Model file for the job. Use its own axes, mm. A direction names the side the tool comes from. Coordinates: 2 decimals unless noted, no trailing zeros. Loops run counter-clockwise (first coordinate to the right, second up) from the corner with the lowest first, then second, coordinate; pieces in that order, holes last.
from build123d import *

# Parameters (mm, degrees)
SKETCH2_W           = 10
SKETCH2_H           = 30
BOSS_EXTRUDE1_DEPTH = 2


with BuildPart() as part:
    # Sketch2 → Boss-Extrude1 (new body)
    with BuildSketch(Plane.XY):
        with Locations((10, -15)):
            Rectangle(SKETCH2_W, SKETCH2_H)
        Polygon((0, 7), (0, 0), (5, 0), (15, 0), (16.8, 0), (16.8, 2.1), (7.2, 4.9), align=None)
        Polygon((8.6, 9.7), (7.2, 4.9), (16.8, 2.1), (18.2, 6.9), align=None)
    extrude(amount=BOSS_EXTRUDE1_DEPTH)


solid = part.part
Q1. Which spindle directions (+Z, -Z, +X, -X, +Y, -Y) get a long thin tool onto all of the face, cutting with end or side? Do faces 4 (the flat face through (7.9, 7.3, 1)), 5 (the flat face through (2, 0, 1)), 6 (the flat face through (16.8, 1, 1)). Say none if no direction does.
Answers:
face 4: +Z, -Z, +Y
face 5: +Z, -Z, -X, -Y
face 6: +Z, -Z, +X, -Y
Q2. Mould opens along X. For faces 1 (the flat face through (3.65, 5.935, 0.986)), 2 (the flat face through (16, 0, 1)), 3 (the flat face through (5, -15, 1)) say: +X half, -X half, draft (parallel to the pull), parting line (faces both ways), or undercut.
Answers:
face 1: undercut
face 2: draft
face 3: -X half
Q3. Drill centre lines: line 1 (X direction, y = -18, z = 1.2); line 2 (Y direction, x = 14.25, z = 0.7); line 3 (Y direction, x = 15.75, z = 1.35). Where is each one in solid material? Low to high.
Answers:
line 1: x = 5 to 15
line 2: y = -30 to 8.05
line 3: y = 0 to 7.61
Q4. Slice it at A-A (z = 0.6). List the corners of the cut face in (x, y).
Answers:
outline: (0, 0) - (5, 0) - (5, -30) - (15, -30) - (15, 0) - (16.8, 0) - (16.8, 2.1) - (18.2, 6.9) - (8.6, 9.7) - (7.2, 4.9) - (0, 7) - close
Q5. Flat gauge pins, fed straight in: P1, Ø0.6, axis at x = 2, z = 1.5, coming from the -Y side; P2, Ø1, axis at y = -12, z = 1, coming from the -X side; P3, Ø0.6, axis at y = -20.5, z = 0.5, coming from the +X side. Where does each tip first touch, or does it go through?
Answers:
P1: stops at y = 0
P2: stops at x = 5
P3: stops at x = 15
Q6. Slice it at B-B (x = 6). List the corners of the cut face in (y, z).
Answers:
outline: (-30, 0) - (5.25, 0) - (5.25, 2) - (-30, 2) - close
Q7. Slice it at C-C (y = -14). List the corners of the cut face in (x, z).
Answers:
outline: (5, 0) - (15, 0) - (15, 2) - (5, 2) - close
